Verification items for the finished model (mm, model axes). Face numbers are marked on the shaded views. A direction names the side the tool comes from. Give positions to 0.01 mm unless a question says otherwise; leave off trailing zeros. Order: outer loops, then holes, each group sorted by start corner. A loop starts at its lowest first (then second) coordinate and runs counter-clockwise, first axis right, second up.
(1) Sectioned sample at B-B on z = 184. Record the cut outline in (x, y), plus the area to 3 significant figures.
(2) Sectioned sample at D-D on z = 123. Record the cut outline in (x, y), plus the area to 3 significant figures.
(3) Access from +Z, -Z, +X, -X, +Y, -Y to the whole of each face (thin tool, end or side, straight path). Record for the marked faces 4 and 5.
(4) Sectioned sample at C-C on x = 208.5. Record the cut outline in (y, z).
(5) Sectioned sample at A-A on y = 43.5. Record the cut outline in (x, z).
(6) Mould release check, pull along Z, two halves, no side actions. Record for the marked faces 1, 2 and 3: pulls with the +Z half, pulls with the -Z half, needs draft (parallel to the pull), parting line crosses it, or undercut.
(7) Scan lines: L1, parallel to Y at x = 19.5, z = 176.5; L2, parallel to Z at x = 92, y = 13; L3, parallel to Y at x = 9.5, z = 212. Record each from-to range of solid material in increasing order.
(8) Gauge pin test, flat ends, axial feed: pin 1 (4 mm diameter, centred on y = 21.5, z = 242, fed in from -X); pin 2 (4 mm diameter, centred on x = 71.5, y = 21, fed in from -Z); pin 3 (10 mm diameter, centred on x = 156, y = 40.5, fed in from -Z). Record the tip position at first contact, or that the pin passes through.
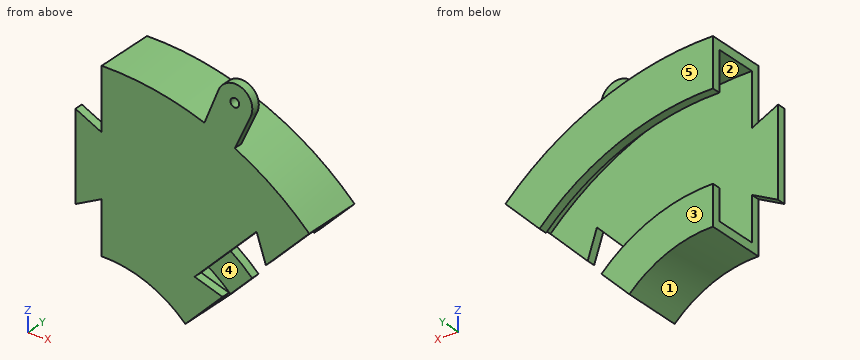
Autodesk Inventor part; units mm, degrees
ref_plane "YZ Plane" through (0, 0, 0) normal (1, 0, 0) x (0, 1, 0)
ref_plane "XZ Plane" through (0, 0, 0) normal (0, 1, 0) x (-1, 0, 0)
ref_plane "XY Plane" through (0, 0, 0) normal (0, 0, 1) x (1, 0, 0)
sketch "Sketch1" plane through (0, 0, 0) normal (0, 1, 0) x (-1, 0, 0)
  circle A0 centre (0, 0) radius 335
  line L0 (335, 0) -> (-335, 0)
  line L1 (0, -335) -> (0, 335)
  line L2 (0, 0) -> (-236.8808, 236.8808)
  line L3 (0, 0) -> (236.8808, -236.8808)
  line L4 (0, 0) -> (236.8808, 236.8808)
  line L5 (0, 0) -> (-236.8808, -236.8808)
  circle A1 centre (0, 0) radius 135
  point P0 (-95.4594, 95.4594)
  point P1 (0, 135)
  dimension "d0" = 670
  dimension "d1" = 45
  dimension "d2" = 45
  dimension "d17" = 200
extrude "Extrusion1" add sketch "Sketch1" along normal blind 70 contours L1 A1 L2 A0
sketch "Sketch2" plane through (95.4594, 0, 95.4594) normal (0.7071068, 0, -0.7071068) x (-0.7071068, 0, -0.7071068)
  line L0 (-190, 60) -> (-10, 60)
  line L1 (-10, 60) -> (-10, 10)
  line L2 (-10, 10) -> (-190, 10)
  line L3 (-190, 10) -> (-190, 60)
  line L4 (-200, 0) -> (0, 0)
  line L5 (-200, 70) -> (0, 70)
  line L6 (-200, 0) -> (-200, 70)
  line L7 (0, 0) -> (0, 70)
  point P0 (135, 0)
  point P1 (0, 35)
  dimension "d6" = 10
  dimension "d7" = 10
  dimension "d8" = 10
  dimension "d9" = 10
sketch3d "3D Sketch1"
  arc A0 (95.4594, 70, 95.4594) -> (0, 70, 135) centre (0, 70, 0) ccw
sweep "Sweep1" cut profiles "Sketch2" path "3D Sketch1" contours L0 L1 L2 L3
sketch "Sketch3" plane through (95.4594, 0, 95.4594) normal (0.7071068, 0, -0.7071068) x (-0.7071068, 0, -0.7071068)
  line L0 (-101.8808, 70) -> (-200, 70)
  line L1 (32.4695, 60) -> (-94.8097, 60)
  line L2 (-145, 70) -> (-45, 70)
  line L3 (-45, 70) -> (-45, 60)
  line L4 (-45, 60) -> (-145, 60)
  line L5 (-145, 60) -> (-145, 70)
  line L6 (-200, 0) -> (-200, 70)
  line L7 (0, 0) -> (0, 70)
  point P0 (135, 0)
  dimension "d16" = 100
  dimension "d18" = 45
sketch3d "3D Sketch2"
  arc A0 (95.4594, 70, 95.4594) -> (0, 70, 135) centre (0, 70, 0) ccw
sweep "Sweep2" cut profiles "Sketch3" path "3D Sketch2"
sketch "Sketch5" plane through (0, 10, 325) normal (0, 1, 0) x (1, 0, 0)
  line L0 (0, 0) -> (0, 180)
  arc A0 (0, 145) -> (127.2792, 197.7208) centre (0, 325) ccw
  line L1 (127.2792, 197.7208) -> (95.4594, 229.5406)
  arc A1 (0, 190) -> (95.4594, 229.5406) centre (0, 325) ccw
  line L2 (0, 190) -> (0, 145)
  arc A2 (0, 45) -> (197.9899, 127.0101) centre (0, 325) ccw
  line L3 (0, 45) -> (0, -10)
  arc A3 (0, -10) -> (236.8808, 88.1192) centre (0, 325) ccw
  line L4 (236.8808, 88.1192) -> (197.9899, 127.0101)
  line L5 (0, 145) -> (-30, 145)
  line L6 (-30, 145) -> (-30, 44.996)
  line L7 (-30, 44.996) -> (0, 44.996)
  line L8 (0, 44.996) -> (0, 145)
  line L9 (0, 190) -> (0, -10)
  line L10 (0, 129.998) -> (-30, 129.998)
  line L11 (-30, 129.998) -> (-30, 59.998)
  line L12 (-30, 59.998) -> (0, 59.998)
  line L13 (0, 59.998) -> (0, 129.998)
  line L14 (0, 44.996) -> (-30, 145) construction
  line L15 (0, 145) -> (-30, 44.996) construction
  line L16 (0, 59.998) -> (-30, 129.998) construction
  line L17 (-30, 59.998) -> (0, 129.998) construction
  line L18 (-15, 94.998) -> (-30, 94.998) construction
  line L19 (-15, 94.998) -> (-30, 94.998) construction
  line L20 (0, 59.998) -> (-30, 44.996)
  line L21 (0, 129.998) -> (-30, 145)
  point P0 (0, 44.996)
  point P1 (0, 59.998)
  dimension "d21" = 30
  dimension "d27" = 70
extrude "Extrusion2" add sketch "Sketch5" against normal blind 10 contours L6 L12 L20 | L12 L6 L10 L0 | L10 L6 L21
sketch "Sketch6" plane through (-30, 10, 280.004) normal (0, 1, 0) x (1, 0, 0)
  line L0 (132.5305, 177.4736) -> (259.8097, 50.1943)
  arc A0 (30, 135.004) -> (132.5305, 177.4736) centre (30, 280.004) ccw
  line L1 (30, 85.002) -> (30, 135.004)
  line L2 (0, 100.004) -> (0, 0)
  line L3 (30, -44.996) -> (30, 15.002)
  arc A1 (30, -44.996) -> (259.8097, 50.1943) centre (30, 280.004) ccw
  arc A2 (30, 100.004) -> (157.2792, 152.7248) centre (30, 280.004) ccw
  line L4 (157.2792, 152.7248) -> (136.066, 131.5116)
  line L5 (136.066, 131.5116) -> (206.7767, 60.8009)
  line L6 (206.7767, 60.8009) -> (227.9899, 82.0141)
  line L7 (227.9899, 82.0141) -> (157.2792, 152.7248)
  arc A3 (30, 100.004) -> (157.2792, 152.7248) centre (30, 280.004) ccw
  arc A4 (30, 0.004) -> (227.9899, 82.0141) centre (30, 280.004) ccw
  line L8 (30, 0.004) -> (30, -54.996)
  arc A5 (30, -54.996) -> (266.8808, 43.1233) centre (30, 280.004) ccw
  line L9 (266.8808, 43.1233) -> (227.9899, 82.0141)
  arc A6 (30, 100.004) -> (157.2792, 152.7248) centre (30, 280.004) ccw
  line L10 (157.2792, 152.7248) -> (125.4594, 184.5446)
  arc A7 (30, 145.004) -> (125.4594, 184.5446) centre (30, 280.004) ccw
  line L11 (30, 145.004) -> (30, 100.004)
  line L12 (167.8858, 142.1182) -> (146.6726, 120.905)
  line L13 (146.6726, 120.905) -> (196.1701, 71.4075)
  line L14 (196.1701, 71.4075) -> (217.3833, 92.6207)
  line L15 (217.3833, 92.6207) -> (167.8858, 142.1182)
  line L16 (167.8858, 142.1182) -> (196.1701, 71.4075) construction
  line L17 (217.3833, 92.6207) -> (146.6726, 120.905) construction
  line L18 (157.2792, 152.7248) -> (206.7767, 60.8009) construction
  line L19 (227.9899, 82.0141) -> (136.066, 131.5116) construction
  line L20 (182.028, 106.7629) -> (171.4214, 96.1563) construction
  line L21 (182.028, 106.7629) -> (171.4214, 96.1563) construction
  line L22 (217.3833, 92.6207) -> (206.7767, 60.8009)
  line L23 (167.8858, 142.1182) -> (136.066, 131.5116)
  line L24 (30, 85.002) -> (0, 100.004)
  line L25 (0, 0) -> (30, 15.002)
  point P0 (207.7219, 63.6364)
  point P1 (217.3833, 92.6207)
  point P2 (167.8858, 142.1182)
  point P3 (205.637, 61.9406)
  dimension "d23" = 30
  dimension "d24" = 70
extrude "Extrusion3" cut sketch "Sketch6" against normal blind 10 contours L0 L14 L5 L12 | L12 L5 L23 | L22 A4 L5 L14 | L22 L5 A4
sketch "Sketch7" plane through (-30, 10, 280.004) normal (0, 1, 0) x (1, 0, 0)
  arc A0 (30, -44.996) -> (259.8097, 50.1943) centre (30, 280.004) ccw
  arc A1 (30, 0.004) -> (227.9899, 82.0141) centre (30, 280.004) ccw
  line L0 (30, 0.004) -> (30, -54.996)
  arc A2 (30, -54.996) -> (266.8808, 43.1233) centre (30, 280.004) ccw
  line L1 (266.8808, 43.1233) -> (227.9899, 82.0141)
  arc A3 (30, -54.996) -> (266.8808, 43.1233) centre (30, 280.004) ccw construction
  line L2 (30, 0.004) -> (266.8808, 43.1233) construction
  line L3 (266.8808, 43.1233) -> (227.9899, 82.0141) construction
  line L4 (266.8808, 43.1233) -> (217.3833, 92.6207) construction
  line L5 (227.9899, 82.0141) -> (227.9899, 82.0141) construction
  line L6 (217.3833, 92.6207) -> (259.8097, 50.1943) construction
  line L7 (227.9899, 82.0141) -> (227.9899, 82.0141) construction
  line L8 (227.9899, 82.0141) -> (227.9899, 82.0141) construction
  line L9 (227.9899, 82.0141) -> (227.9899, 82.0141) construction
  line L10 (227.9899, 82.0141) -> (39.9698, -54.8476) construction
  line L11 (143.7771, 20.7148) -> (196.6229, -99.7168) construction
  circle A4 centre (181.9243, -66.2198) radius 20
  line L12 (163.3808, -73.7121) -> (147.2566, -33.8047)
  line L13 (200.0777, -57.8259) -> (181.9244, -18.5659)
  circle A5 centre (181.9243, -66.2198) radius 5
  point P0 (181.9244, -18.5659)
  point P1 (147.2566, -33.8047)
  dimension "d28" = 40
  dimension "d31" = 10
extrude "Extrusion4" add sketch "Sketch7" against normal blind 10 contours A2 L13 A4 L12 | A4
properties part number "Carousel Fixed Track" material "PLA Plastic"
Ans:
1. outline: (-30, 0) - (-22, 0) - (-22, 10) - (-30, 10) - close; (0, 0) - (141.57, 0) - (141.57, 10) - (0, 10) - close
1. area: 1,500 mm2
2. outline: (55.64, 0) - (123, 0) - (123, 10) - (76.79, 10) - (76.79, 60) - (123, 60) - (123, 70) - (55.64, 70) - close
2. area: 2,400 mm2
3. face 4: +X
3. face 5: +Z, -Z, +X, -X, +Y
4. outline: (0, 208.5) - (10, 208.5) - (10, 249.3) - (60, 249.3) - (60, 208.5) - (70, 208.5) - (70, 262.21) - (0, 262.21) - close
5. outline: (0, 135) arc R135 cw to (95.46, 95.46) - (102.53, 102.53) arc R145 ccw to (0, 145) - close; (0, 325) arc R325 cw to (229.81, 229.81) - (236.88, 236.88) arc R335 ccw to (0, 335) - close
6. face 1: pulls with the -Z half
6. face 2: undercut
6. face 3: needs draft
7. L1: y = 0 to 10, 60 to 70
7. L2: z = 98.8 to 112.08, 311.71 to 322.12
7. L3: y = 0 to 10
8. pin 1: stops at x = 214.68
8. pin 2: stops at z = 113.24
8. pin 3: stops at z = 282.32
